Check sheet for the modelled part. Datum: model origin and axes. Units: mm. Face numbers are marked on the shaded views. A direction names the side the tool comes from. Give positions to 0.01 mm unless a question says otherwise; leave off trailing zeros. Order: outer loops, then holes, each group sorted by start corner. A loop starts at its lowest first (then second) coordinate and runs counter-clockwise, first axis right, second up.
```python
from build123d import *

# Parameters (mm, degrees)
F0_R     = 10
F0_R_2   = 1.25
F1_DEPTH = 2.5
F2_R     = 3.95
F2_R_2   = 1.25
F3_DEPTH = 6.3
F2_R_3   = 5.75
F4_DEPTH = 0.5
F5_R     = 0.5


with BuildPart() as f1:
    # F0 (on Top) → F1 (new body)
    with BuildSketch(Plane.XY):
        Circle(F0_R)
        Circle(F0_R_2, mode=Mode.SUBTRACT)
    extrude(amount=F1_DEPTH)

    # F2 (on face) → F3 (join)
    with BuildSketch(Plane.XY.offset(2.5)):
        Circle(F2_R)
        Circle(F2_R_2, mode=Mode.SUBTRACT)
    extrude(amount=F3_DEPTH)

    # F2 (on face) → F4 (join)
    with BuildSketch(Plane.XY.offset(2.5)):
        Circle(F2_R_3)
        Circle(F2_R, mode=Mode.SUBTRACT)
    extrude(amount=F4_DEPTH)

    # F5
    f5_edges = [f1.edges().sort_by_distance(p)[0] for p in [
        (-10, 0, 0),
        (-10, 0, 2.5),
    ]]
    fillet(f5_edges, radius=F5_R)


solid = f1.part
```
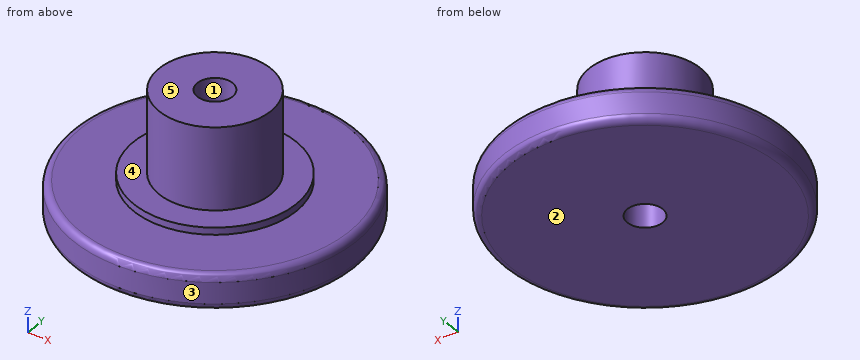
(1) Release check for a two-part mould opening along Y. For the marked faces 1, 2 and 3 record: released by +Y, released by -Y, zero draft, split by the parting line, or undercut.
(2) Go/stop test with flat-tipped pins: P1, Ø1, axis at x = 0, y = -7, coming from the +Z side; P2, Ø1.5, axis at x = 0, y = 0, coming from the +Z side. Record where each tip stops, or that it passes through.
(3) Sectioned sample at C-C (z = 3.25). Enter the section's corners in (x, y), plus the area to 3 significant figures.
(4) Sectioned sample at A-A (y = 0). Enter the section's corners in (x, z).
(5) Tool access check on the marked faces 4 and 5. Record the directions out of +Z, -Z, +X, -X, +Y, -Y that give a thin tool (end or side, any length) a straight path to the whole face; none if there is none.
(6) Thickness scan on L1, parallel to Y at x = 0, z = 3.25; L2, parallel to Z at x = 6.5, y = 1; L3, parallel to Z at x = 4, y = -2.25. Record the ranges inside material, lowest first.
Values follow:
1. face 1: undercut
1. face 2: zero draft
1. face 3: split by the parting line
2. P1: stops at z = 2.5
2. P2: passes through
3. outline: circle Ø7.9 at (0, 0); hole circle Ø2.5 at (0, 0)
3. area: 44.1 mm2
4. outline: (-10, 0.5) arc R0.5 ccw to (-9.5, 0) - (-1.25, 0) - (-1.25, 8.8) - (-3.95, 8.8) - (-3.95, 3) - (-5.75, 3) - (-5.75, 2.5) - (-9.5, 2.5) arc R0.5 ccw to (-10, 2) - close; (1.25, 0) - (9.5, 0) arc R0.5 ccw to (10, 0.5) - (10, 2) arc R0.5 ccw to (9.5, 2.5) - (5.75, 2.5) - (5.75, 3) - (3.95, 3) - (3.95, 8.8) - (1.25, 8.8) - close
5. face 4: +Z
5. face 5: +Z, +X, -X, +Y, -Y
6. L1: y = -3.95 to -1.25, 1.25 to 3.95
6. L2: z = 0 to 2.5
6. L3: z = 0 to 3
